Can you work these out from the model? Positions are in its coordinate system, mm. Face numbers are marked on the shaded views. Give positions to 0.01 mm unless a question says otherwise; leave off trailing zeros. Order: outer loops, then holes, each group sorted by start corner. A loop starts at its lowest first (then second) coordinate and runs counter-clockwise, first axis right, second up. Notation, with made-up numbers: (40.25, 32) - (92.25, 32) arc R23 ccw to (92.25, 65) - close; hole circle Ø5 at (78, 53.25). An arc over 180 degrees is marked (long way). One line per question, with ' | ' between items.
```python
from build123d import *

# Parameters (mm, degrees)
ESQUISSE1_W             = 69.2
ESQUISSE1_H             = 50
BOSS_EXTRU_1_DEPTH      = 2.2
ENL_V_MAT_EXTRU_1_DEPTH = 1


with BuildPart() as part:
    # Esquisse1 → Boss.-Extru.1 (new body)
    with BuildSketch(Plane.XY):
        Rectangle(ESQUISSE1_W, ESQUISSE1_H)
    extrude(amount=BOSS_EXTRU_1_DEPTH)

    # Esquisse2 → Enlèv. mat.-Extru.1 (cut)
    with BuildSketch(Plane.XY.offset(2.2)):
        Polygon((34.6, 20.704314338), (31.104320123, 20.704314338), (31.104320123, 23.495586326), (-33.095389285, 23.495586326), (-33.095389285, 8.25), (-34.510836618, 8.25), (-34.6, 8.25), (-34.6, -8.25), (-33.095389285, -8.25), (-33.095389285, -23.5), (31.104320123, -23.5), (31.104320123, -14.404258976), (34.6, -14.404258976), align=None)
    extrude(amount=-ENL_V_MAT_EXTRU_1_DEPTH, mode=Mode.SUBTRACT)


solid = part.part
```
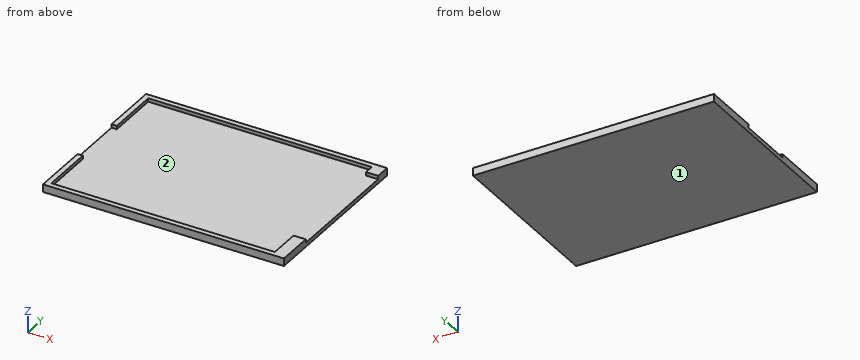
(1) If we mould it in two halves opening along Y, with no side actions, what happens to the marked faces 1 and 2? For each: released by +Y, released by -Y, zero draft, split by the parting line, or undercut.
Answer below:
face 1: zero draft | face 2: undercut
(2) Imagine slicing it at C-C (x = 18). List the corners of the cut face in (y, z) for me.
Answer below:
outline: (-25, 0) - (25, 0) - (25, 2.2) - (23.5, 2.2) - (23.5, 1.2) - (-23.5, 1.2) - (-23.5, 2.2) - (-25, 2.2) - close
(3) Imagine slicing it at A-A (z = 1.65). List the corners of the cut face in (x, y) for me, and give its area (3 significant figures).
Answer below:
outline: (-34.6, -25) - (34.6, -25) - (34.6, -14.4) - (31.1, -14.4) - (31.1, -23.5) - (-33.1, -23.5) - (-33.1, -8.25) - (-34.6, -8.25) - close; (-34.6, 8.25) - (-33.1, 8.25) - (-33.1, 23.5) - (31.1, 23.5) - (31.1, 20.7) - (34.6, 20.7) - (34.6, 25) - (-34.6, 25) - close | area: 295 mm^2
(4) Will these pins go through, and if not, where does the flat tip stop? pin 1 (1.1 mm diameter, centred on y = -13.5, z = 2, fed in from +X); pin 2 (23.5 mm diameter, centred on x = -12, y = -8, fed in from +Z).
Answer below:
pin 1: x = -33.1 | pin 2: z = 1.2
(5) Imagine slicing it at D-D (y = -10.5). List the corners of the cut face in (x, z) for me.
Answer below:
outline: (-34.6, 0) - (34.6, 0) - (34.6, 1.2) - (-33.1, 1.2) - (-33.1, 2.2) - (-34.6, 2.2) - close
(6) If I drill on line 1 (Y direction, x = 22, z = 1.8); line 2 (X direction, y = -15, z = 1.65); line 3 (Z direction, x = -29.5, y = 15.5), over which ranges is the centre line in solid material (lowest first)?
Answer below:
line 1: -25 to -23.5, 23.5 to 25 | line 2: -34.6 to -33.1, 31.1 to 34.6 | line 3: 0 to 1.2
(7) Imagine slicing it at B-B (y = -20). List the corners of the cut face in (x, z) for me, and give its area (3 significant figures).
Answer below:
outline: (-34.6, 0) - (34.6, 0) - (34.6, 2.2) - (31.1, 2.2) - (31.1, 1.2) - (-33.1, 1.2) - (-33.1, 2.2) - (-34.6, 2.2) - close | area: 88.0 mm^2
